Build history of the part. All positions in model axes, mm. Face numbers are marked on the shaded views. A direction names the side the tool comes from. Give positions to 0.01 mm unless a question says otherwise; leave off trailing zeros. Write each loop counter-clockwise with the first axis right and the second up, starting at its lowest first coordinate (ties: lowest second). Pieces come first, ordered by that corner, then holes. Notation, with made-up numbers: M 41,-27.75 L 99,-27.75 A8 ccw 99,-21.75 Z; hole C 80.25,24 d1. An arc over 180 degrees is marked long. Return JSON: item names as keys, results as strings. Group by question number.
Q1. Band-saw the part on D-D, the plane z = 9. Give the cut face in (x, y), then the cut area to 3 significant figures.
Q2. Flat gauge pins, fed straight in: pin 1 Ø1.5 at (y, z) = (5.5, 6) entering from +X; pin 2 Ø1.5 at (y, z) = (6, -12) entering from -X; pin 3 Ø3 at (x, y) = (0, 8) entering from -Z. Where does each tip first touch, or does it go through?
Q3. Band-saw the part on B-B, the plane z = 0. Give the cut face in (x, y), then the cut area to 3 significant figures.
Q4. Band-saw the part on A-A, the plane x = 0. Give the cut face in (y, z), then the cut area to 3 significant figures.
Q5. Band-saw the part on C-C, the plane y = 11. Give the cut face in (x, z).
Q6. Wall check: probe 1 along Z at (x, y) = (0, 3.5); probe 2 along Y at (x, z) = (10, -14.5); probe 3 along Z at (x, y) = (4.5, 2.25). Give the ranges that are in metal, low to high.
Q7. Tool access for the marked faces 4 and 5: list every direction of +Z, -Z, +X, -X, +Y, -Y with a clear straight run to the whole face (end or side of a thin tool).
Q8. Pull direction Z, two halves, no side cores. Call the marked faces 1, 2 and 3: +Z half, -Z half, draft (parallel to the pull), parting line (faces both ways), or undercut.
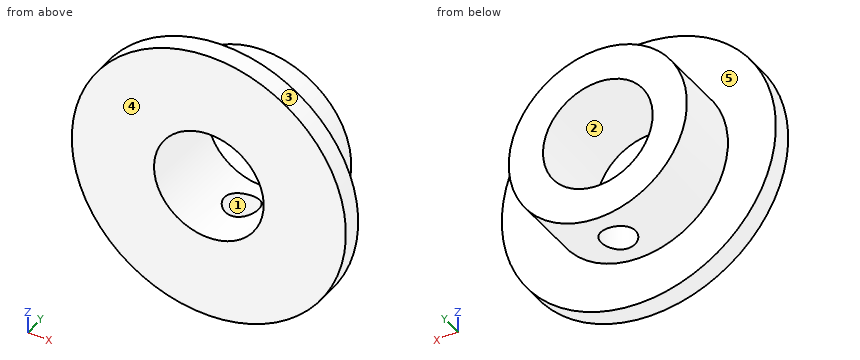
from build123d import *

# Parameters (mm, degrees)
SKETCH1_R           = 20
SKETCH1_R_2         = 8
BOSS_EXTRUDE1_DEPTH = 3
SKETCH2_R           = 13
SKETCH2_R_2         = 8
BOSS_EXTRUDE2_DEPTH = 10
SKETCH3_R           = 2.5
CUT_EXTRUDE1_DEPTH  = 32.128764833


with BuildPart() as part:
    # Sketch1 → Boss-Extrude1 (new body)
    with BuildSketch(Plane(origin=(0, 0, 0), x_dir=(1, 0, 0), z_dir=(0, 1, 0))):
        with Locations(Location((0, 0, 0), (0, 0, 270))):
            Circle(SKETCH1_R)
        with Locations(Location((0, 0, 0), (0, 0, 270))):
            Circle(SKETCH1_R_2, mode=Mode.SUBTRACT)
    extrude(amount=BOSS_EXTRUDE1_DEPTH)

    # Sketch2 → Boss-Extrude2 (add)
    with BuildSketch(Plane(origin=(0, 3, 0), x_dir=(1, 0, 0), z_dir=(0, 1, 0))):
        with Locations(Location((0, 0, 0), (0, 0, 270))):
            Circle(SKETCH2_R)
        with Locations(Location((0, 0, 0), (0, 0, 270))):
            Circle(SKETCH2_R_2, mode=Mode.SUBTRACT)
    extrude(amount=BOSS_EXTRUDE2_DEPTH)

    # Sketch3 → Cut-Extrude1 (cut, through all)
    with BuildSketch(Plane.XY):
        with Locations(Location((0, 8, 0), (0, 0, 90))):
            Circle(SKETCH3_R)
    extrude(amount=-CUT_EXTRUDE1_DEPTH, mode=Mode.SUBTRACT)


solid = part.part
From the geometry:
{
 "1": {"outline": "M -17.86,0 L 17.86,0 L 17.86,3 L 9.38,3 L 9.38,13 L -9.38,13 L -9.38,3 L -17.86,3 Z", "area": "295 mm^2"},
 "2": {"pin 1": "stops at x = 11.89", "pin 2": "stops at x = -6.51", "pin 3": "stops at z = 7.86"},
 "3": {"outline": "M -20,0 L -8,0 L -8,13 L -13,13 L -13,3 L -20,3 Z; M 8,0 L 20,0 L 20,3 L 13,3 L 13,13 L 8,13 Z", "area": "172 mm^2"},
 "4": {"outline": "M 0,-20 L 3,-20 L 3,-13 L 5.5,-13 L 5.5,-8 L 0,-8 Z; M 0,8 L 13,8 L 13,13 L 3,13 L 3,20 L 0,20 Z; M 10.5,-13 L 13,-13 L 13,-8 L 10.5,-8 Z", "area": "147 mm^2"},
 "5": {"outline": "C 0,0 d26; hole C 0,0 d16"},
 "6": {"probe 1": "z = -13 to -8, 8 to 13", "probe 2": "y = 0 to 3", "probe 3": "z = -19.49 to -6.61, 6.61 to 19.49"},
 "7": {"face 4": "+Z, -Z, +X, -X, -Y", "face 5": "+Y"},
 "8": {"face 1": "draft", "face 2": "undercut", "face 3": "parting line"}
}
